Geometry: final body of the model. Coordinates: model frame, mm. Face numbers are marked on the shaded views. A direction names the side the tool comes from. Give positions to 0.01 mm unless a question says otherwise; leave off trailing zeros. Write each loop counter-clockwise with the first axis right and the second up, starting at its lowest first coordinate (ties: lowest second). Pieces come first, ordered by that corner, then holes.
Q1. Reachability of the marked faces 1, 2, 3 and 4 from +Z, -Z, +X, -X, +Y, -Y: full face, straight path, thin tool, end or side. Return the list, or none.
Q2. Cut plane C-C on x = 5.5. Return the cut outline in (y, z).
Q3. Draft query along X for the marked faces 5, 6 and 7. Return one class per face: pulls with the +X half, pulls with the -X half, needs draft (parallel to the pull), parting line crosses it, or undercut.
Q4. Pin query (flat end, axial travel): pin 1 (1 mm diameter, centred on x = -2.5, z = 2.5, fed in from +Y); pin 2 (2.5 mm diameter, centred on y = -27, z = 2.5, fed in from -X); pin 3 (1 mm diameter, centred on y = 20.5, z = 1.5, fed in from +X); pin 4 (1.5 mm diameter, centred on x = 18.5, z = 2.5, fed in from +Y). Return the tip coordinate at first contact, or that it passes through.
Q5. Cut plane D-D on x = 38.5. Return the cut outline in (y, z), plus the area to 3 significant figures.
Q6. Line query: L1, parallel to X at y = -25, z = 1.3; L2, parallel to Y at x = 31, z = 0.85; L3, parallel to X at y = 3, z = 3. Output: solid intervals per line, ascending.
Q7. Cut plane B-B on y = 0. Return the cut outline in (x, z), plus the area to 3 significant figures.
Q8. Cut plane A-A on y = 52. Return the cut outline in (x, z).
```python
from build123d import *

# Parameters (mm, degrees)
BOSS_EXTRUDE1_DEPTH = 5.08
SKETCH2_R           = 15.5
SKETCH2_R_2         = 2
SKETCH2_W           = 7
SKETCH2_H           = 6
SKETCH2_W_2         = 5.08
SKETCH2_H_2         = 5
CUT_EXTRUDE1_DEPTH  = 6.08
SKETCH4_W           = 5.08
SKETCH4_H           = 10
CUT_EXTRUDE2_DEPTH  = 6.08
SKETCH5_R           = 7.5
BOSS_EXTRUDE2_DEPTH = 5.08
SKETCH6_W           = 5.08
SKETCH6_H           = 12
SKETCH6_W_2         = 8
SKETCH6_H_2         = 5.08
CUT_EXTRUDE3_DEPTH  = 6.08
FILLET1_R           = 10


with BuildPart() as part:
    # Sketch1 → Boss-Extrude1 (new body)
    with BuildSketch(Plane.XY):
        Polygon((32.5, 19), (43, 10), (43, -10), (32.5, -19), (32.5, -29), (-33.5, -29), (-33.5, 31), (32.5, 31), align=None)
    extrude(amount=BOSS_EXTRUDE1_DEPTH)

    # Sketch2 → Cut-Extrude1 (cut, through all)
    with BuildSketch(Plane(origin=(0, 0, 0), x_dir=(-1, 0, 0), z_dir=(0, 0, -1))):
        Circle(SKETCH2_R)
        with Locations((15.5, -15.5)):
            Circle(SKETCH2_R_2)
        with Locations((-15.5, -15.5)):
            Circle(SKETCH2_R_2)
        with Locations((-15.5, 15.5)):
            Circle(SKETCH2_R_2)
        with Locations((15.5, 15.5)):
            Circle(SKETCH2_R_2)
        with Locations((-11.5, -26)):
            Rectangle(SKETCH2_W, SKETCH2_H)
        with Locations((2.5, -26)):
            Rectangle(SKETCH2_W, SKETCH2_H)
        with Locations((-38.04, 0)):
            Rectangle(SKETCH2_W_2, SKETCH2_H_2)
    extrude(amount=-CUT_EXTRUDE1_DEPTH, mode=Mode.SUBTRACT)

    # Sketch4 → Cut-Extrude2 (cut, through all)
    with BuildSketch(Plane.XY.offset(5.08)):
        with Locations((29.96, 1)):
            Rectangle(SKETCH4_W, SKETCH4_H)
        with Locations((29.96, -24)):
            Rectangle(SKETCH4_W, SKETCH4_H)
        with Locations((29.96, 26)):
            Rectangle(SKETCH4_W, SKETCH4_H)
        with Locations((-30.96, -24)):
            Rectangle(SKETCH4_W, SKETCH4_H)
        with Locations((-30.96, 1)):
            Rectangle(SKETCH4_W, SKETCH4_H)
        with Locations((-30.96, 26)):
            Rectangle(SKETCH4_W, SKETCH4_H)
    extrude(amount=-CUT_EXTRUDE2_DEPTH, mode=Mode.SUBTRACT)

    # Sketch5 → Boss-Extrude2 (add)
    with BuildSketch(Plane.XY.offset(5.08)):
        Polygon((-8, 63), (7, 63), (7, 31), (-8, 31), (-8, 41), (-33.5, 41), (-33.5, 63), align=None)
        with Locations((-17.5, 52)):
            Circle(SKETCH5_R, mode=Mode.SUBTRACT)
    extrude(amount=-BOSS_EXTRUDE2_DEPTH)

    # Sketch6 → Cut-Extrude3 (cut, through all)
    with BuildSketch(Plane.XY.offset(5.08)):
        with Locations((-30.96, 57)):
            Rectangle(SKETCH6_W, SKETCH6_H)
        with Locations((4.5, 45.54)):
            Rectangle(SKETCH6_W_2, SKETCH6_H_2)
    extrude(amount=-CUT_EXTRUDE3_DEPTH, mode=Mode.SUBTRACT)

    # Fillet1
    fillet1_edges = [part.edges().sort_by_distance(p)[0] for p in [
        (7, 63, 2.54),
    ]]
    fillet(fillet1_edges, radius=FILLET1_R)


solid = part.part
```
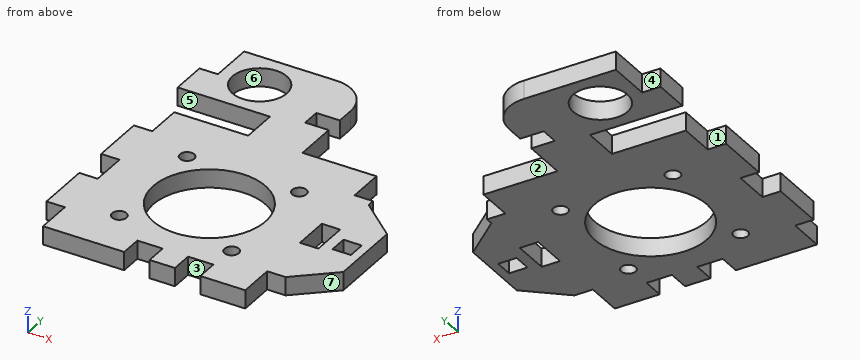
Data:
1. face 1: +Z, -Z, -X
1. face 2: +Z, -Z, +X, +Y
1. face 3: +Z, -Z, -Y
1. face 4: +Z, -Z, -X, +Y
2. outline: (-29, 0) - (-14.49, 0) - (-14.49, 5.08) - (-29, 5.08) - close; (14.49, 0) - (43, 0) - (43, 5.08) - (14.49, 5.08) - close; (48.08, 0) - (58.27, 0) - (58.27, 5.08) - (48.08, 5.08) - close
3. face 5: needs draft
3. face 6: undercut
3. face 7: pulls with the +X half
4. pin 1: stops at y = 63
4. pin 2: stops at x = -28.42
4. pin 3: stops at x = 32.5
4. pin 4: stops at y = 31
5. outline: (-13.86, 0) - (-2.5, 0) - (-2.5, 5.08) - (-13.86, 5.08) - close; (2.5, 0) - (13.86, 0) - (13.86, 5.08) - (2.5, 5.08) - close
5. area: 115 mm2
6. L1: x = -28.42 to -6, 1 to 8, 15 to 27.42
6. L2: y = -19 to -4, 6 to 21
6. L3: x = -28.42 to -15.21, 15.21 to 27.42, 32.5 to 43
7. outline: (-28.42, 0) - (-15.5, 0) - (-15.5, 5.08) - (-28.42, 5.08) - close; (15.5, 0) - (27.42, 0) - (27.42, 5.08) - (15.5, 5.08) - close; (32.5, 0) - (35.5, 0) - (35.5, 5.08) - (32.5, 5.08) - close; (40.58, 0) - (43, 0) - (43, 5.08) - (40.58, 5.08) - close
7. area: 154 mm2
8. outline: (-28.42, 0) - (-25, 0) - (-25, 5.08) - (-28.42, 5.08) - close; (-10, 0) - (7, 0) - (7, 5.08) - (-10, 5.08) - close
